```python
from build123d import *

# Parameters (mm, degrees)
SKETCH1_W                 = 42.3
SKETCH1_H                 = 42.3
BOSS_EXTRUDE1_DEPTH       = 34
SKETCH2_R                 = 18
BOSS_EXTRUDE2_DEPTH       = 35
SKETCH3_R                 = 11
BOSS_EXTRUDE3_DEPTH       = 2
SKETCH4_R                 = 3
BOSS_EXTRUDE4_DEPTH       = 16
CUT_EXTRUDE1_DEPTH        = 12
CHAMFER1_SIZE             = 5
M3X0_5_TAPPED_HOLE1_D     = 2.5
M3X0_5_TAPPED_HOLE1_DEPTH = 7.5
M3X0_5_TAPPED_HOLE1_TIP   = 0.751075774


with BuildPart() as part:
    # Sketch1 → Boss-Extrude1 (new body)
    with BuildSketch(Plane.XY):
        Rectangle(SKETCH1_W, SKETCH1_H)
    extrude(amount=BOSS_EXTRUDE1_DEPTH)

    # Sketch2 → Boss-Extrude2 (add)
    with BuildSketch(Plane.XY.offset(34)):
        Circle(SKETCH2_R)
    extrude(amount=BOSS_EXTRUDE2_DEPTH)

    # Sketch3 → Boss-Extrude3 (add)
    with BuildSketch(Plane.XY.offset(69)):
        Circle(SKETCH3_R)
    extrude(amount=BOSS_EXTRUDE3_DEPTH)

    # Sketch4 → Boss-Extrude4 (add)
    with BuildSketch(Plane.XY.offset(71)):
        Circle(SKETCH4_R)
    extrude(amount=BOSS_EXTRUDE4_DEPTH)

    # Sketch5 → Cut-Extrude1 (cut)
    with BuildSketch(Plane.XY.offset(87)):
        with BuildLine():
            Line((-2, 2.236067977), (-2, -2.236067977))
            ThreePointArc((-2, -2.236067977), (-3, 0), (-2, 2.236067977))
        make_face()
    extrude(amount=-CUT_EXTRUDE1_DEPTH, mode=Mode.SUBTRACT)

    # Chamfer1
    chamfer1_edges = [part.edges().sort_by_distance(p)[0] for p in [
        (-21.15, -21.15, 17),
        (21.15, -21.15, 17),
        (21.15, 21.15, 17),
        (-21.15, 21.15, 17),
    ]]
    chamfer(chamfer1_edges, length=CHAMFER1_SIZE)

    # M3x0.5 Tapped Hole1
    with Locations(Plane.XY.offset(69)):
        with Locations((-9.899494937, 9.899494937), (9.899494937, 9.899494937), (9.899494937, -9.899494937), (-9.899494937, -9.899494937)):
            Hole(M3X0_5_TAPPED_HOLE1_D / 2, depth=M3X0_5_TAPPED_HOLE1_DEPTH)
            with Locations((0, 0, -(M3X0_5_TAPPED_HOLE1_DEPTH + M3X0_5_TAPPED_HOLE1_TIP / 2))):  # 118° drill point
                Cone(0, M3X0_5_TAPPED_HOLE1_D / 2, M3X0_5_TAPPED_HOLE1_TIP, mode=Mode.SUBTRACT)


solid = part.part
```
The model under review builds one solid part; all positions refer to its coordinate system, in mm. A direction names the side the tool comes from. Round coordinates to 2 decimals unless told otherwise and drop trailing zeros. Write each loop counter-clockwise with the first axis right and the second up, starting at its lowest first coordinate (ties: lowest second). Pieces come first, ordered by that corner, then holes. Notation, with made-up numbers: (10, -19.5) - (66, -19.5) arc R21 ccw to (66, 8.5) - close; hole circle Ø7 at (10, -1). An arc over 180 degrees is marked (long way). One line per question, with ' | ' between items.
Item 1: The part is to be moulded in two halves that separate along Y. For faces 1 (the face through (-8, -8, 69)), 2 (the face through (-11.054, -10.378, 65.198)), 3 (the face through (18.7, -18.6, 16.8)), say which applies: pulls with the +Y half, pulls with the -Y half, needs draft (parallel to the pull), parting line crosses it, or undercut.
Resolved:
face 1: needs draft | face 2: undercut | face 3: pulls with the -Y half
Item 2: To check wall thickness, follow probe 1 along Z at (x, y) = (-14.5, -11); probe 2 along Z at (x, y) = (-1.5, -14); probe 3 along Y at (x, z) = (-3.5, 61). State the ranges of each line that lie inside material, in increasing order.
Resolved:
probe 1: z = 0 to 34 | probe 2: z = 0 to 69 | probe 3: y = -17.66 to 17.66
Item 3: Add section B-B, the plane z = 29. Give the boundary of the cut face in (x, y).
Resolved:
outline: (-21.15, -16.15) - (-16.15, -21.15) - (16.15, -21.15) - (21.15, -16.15) - (21.15, 16.15) - (16.15, 21.15) - (-16.15, 21.15) - (-21.15, 16.15) - close
Item 4: Add section A-A, the plane x = 0. Give the boundary of the cut face in (y, z).
Resolved:
outline: (-21.15, 0) - (21.15, 0) - (21.15, 34) - (18, 34) - (18, 69) - (11, 69) - (11, 71) - (3, 71) - (3, 87) - (-3, 87) - (-3, 71) - (-11, 71) - (-11, 69) - (-18, 69) - (-18, 34) - (-21.15, 34) - close
Item 5: Add section C-C, the plane y = 0. Give the boundary of the cut face in (x, z).
Resolved:
outline: (-21.15, 0) - (21.15, 0) - (21.15, 34) - (18, 34) - (18, 69) - (11, 69) - (11, 71) - (3, 71) - (3, 87) - (-2, 87) - (-2, 75) - (-3, 75) - (-3, 71) - (-11, 71) - (-11, 69) - (-18, 69) - (-18, 34) - (-21.15, 34) - close
Item 6: Add section D-D, the plane x = -7. Give the boundary of the cut face in (y, z).
Resolved:
outline: (-21.15, 0) - (21.15, 0) - (21.15, 34) - (16.58, 34) - (16.58, 69) - (8.49, 69) - (8.49, 71) - (-8.49, 71) - (-8.49, 69) - (-16.58, 69) - (-16.58, 34) - (-21.15, 34) - close
Item 7: For faces 4 (the face through (0, 0, 0)), 5 (the face through (10.17, -11.12, 65.2)), list the 3-axis set-ups (+Z, -Z, +X, -X, +Y, -Y) from which the entire face can be reached by the end or side of a thin tool; tool diameter is ignored.
Resolved:
face 4: -Z, +X, -X, +Y, -Y | face 5: +Z
Item 8: For P1, Ø8, axis at y = -1, z = 71.5, coming from the -X side; P2, Ø2, axis at x = -9.9, y = 9.9, coming from the +Z side; P3, Ø8, axis at x = 7.5, z = 66.5, coming from the -Y side, all flat-tipped, find the tip position at first contact; note any pin that passes through.
Resolved:
P1: stops at x = -18 | P2: stops at z = 61.35 | P3: stops at y = -17.66
